Read the model definition and answer for the solid it produces. Units are mm, in the model's axes. Face numbers are marked on the shaded views. Coordinates: 2 decimals unless noted, no trailing zeros. Write each loop counter-clockwise with the first axis right and the second up, starting at its lowest first coordinate (ties: lowest second). Pieces come first, ordered by that corner, then holes.
1) Find the intervals of material crossed by line 1 (X direction, y = 7, z = 0); line 2 (Z direction, x = 1, y = 17.5); line 3 (Y direction, x = 53, z = 42), in increasing order.
2) The part is cut by section A-A (z = 0). Determine the outline of the cut face in (x, y).
3) Determine the mould class of the marked faces 1 and 2 for opening direction X: +X half, -X half, draft (parallel to the pull), parting line (faces both ways), or undercut.
4) The part is cut by section B-B (x = 0). Determine the outline of the cut face in (y, z).
5) Each of these flat-tipped pins is pushed along its axis until it touches: pin 1 Ø4 at (y, z) = (7, 14.5) entering from -X; pin 2 Ø6 at (y, z) = (17, 47) entering from +X; pin 3 Ø5 at (x, y) = (45.5, 17) entering from -Z. Where does it stop, or does it pass through?
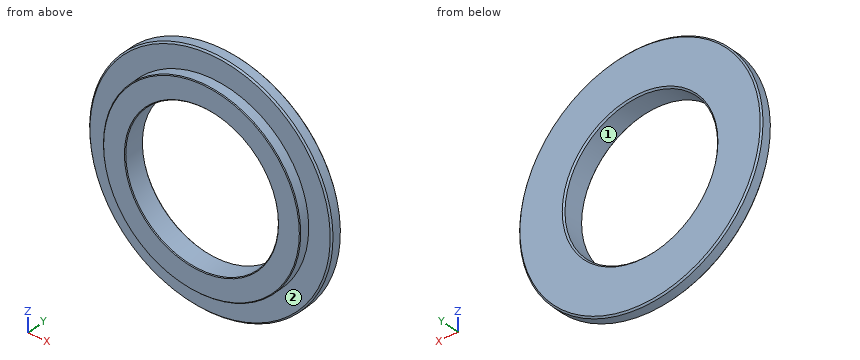
from build123d import *

# Parameters (mm, degrees)
SKETCH_1_W      = 80.5
SKETCH_1_H      = 8
SKETCH_2_R      = 65.25
EXTRUDE_1_DEPTH = 7
HOLE_WIZARD_3_D = 101
CHAMFER_1_SIZE  = 0.5
CHAMFER_2_SIZE2 = 1.000000001
CHAMFER_2_SIZE  = 0.999999999


with BuildPart() as part:
    # 草圖1 → 旋轉1 (revolve)
    with BuildSketch(Plane.XY, mode=Mode.PRIVATE) as revolve_1_sk:
        with Locations((40.25, 15)):
            Rectangle(SKETCH_1_W, SKETCH_1_H)
    revolve(revolve_1_sk.sketch.rotate(Axis((0, 19, 0), (0, -1, 0)), 270), axis=Axis((0, 19, 0), (0, -1, 0)))

    # 草圖2 → 填料-伸長1 (add)
    with BuildSketch(Plane.XZ.offset(-11)):
        with Locations(Location((0, 0, 0), (0, 0, 90))):
            Circle(SKETCH_2_R)
    extrude(amount=EXTRUDE_1_DEPTH)

    # 鑽孔3 (through all)
    with Locations(Plane(origin=(0, 4, 0), x_dir=(-1, 0, 0), z_dir=(0, -1, 0))):
        with Locations((0, 0)):
            Hole(HOLE_WIZARD_3_D / 2)

    # 導角1
    chamfer_1_edges = [part.edges().sort_by_distance(p)[0] for p in [
        (0, 4, -65.25),
        (-50.5, 4, 0),
    ]]
    chamfer(chamfer_1_edges, length=CHAMFER_1_SIZE)

    # 導角2
    chamfer_2_edges = [part.edges().sort_by_distance(p)[0] for p in [
        (-50.5, 19, 0),
        (0, 11, 80.5),
        (0, 19, 80.5),
    ]]
    chamfer(chamfer_2_edges, length=CHAMFER_2_SIZE, length2=CHAMFER_2_SIZE2)


solid = part.part
Reported:
1. line 1: x = -65.25 to -50.5, 50.5 to 65.25
1. line 2: z = -80.49 to -50.49, 50.49 to 80.49
1. line 3: y = 11 to 19
2. outline: (-80.5, 12) - (-79.5, 11) - (-65.25, 11) - (-65.25, 4.5) - (-64.75, 4) - (-51, 4) - (-50.5, 4.5) - (-50.5, 18) - (-51.5, 19) - (-79.5, 19) - (-80.5, 18) - close; (50.5, 4.5) - (51, 4) - (64.75, 4) - (65.25, 4.5) - (65.25, 11) - (79.5, 11) - (80.5, 12) - (80.5, 18) - (79.5, 19) - (51.5, 19) - (50.5, 18) - close
3. face 1: undercut
3. face 2: draft
4. outline: (4, -64.75) - (4.5, -65.25) - (11, -65.25) - (11, -79.5) - (12, -80.5) - (18, -80.5) - (19, -79.5) - (19, -51.5) - (18, -50.5) - (4.5, -50.5) - (4, -51) - close; (4, 51) - (4.5, 50.5) - (18, 50.5) - (19, 51.5) - (19, 79.5) - (18, 80.5) - (12, 80.5) - (11, 79.5) - (11, 65.25) - (4.5, 65.25) - (4, 64.75) - close
5. pin 1: stops at x = -64.04
5. pin 2: stops at x = 67.41
5. pin 3: stops at z = -68.05
